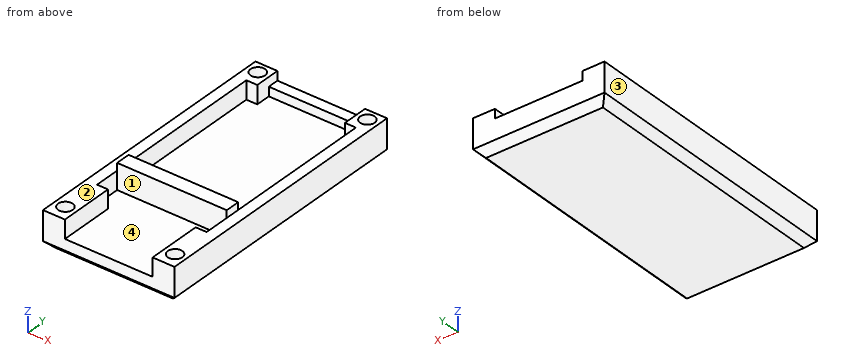
```python
from build123d import *

# Parameters (mm, degrees)
F1_DEPTH  = 37
F2_W      = 12
F2_H      = 1.25
F3_DEPTH  = 2
F5_DEPTH  = 2.5
F7_W      = 15
F7_H      = 2
F8_DEPTH  = 3.5
F9_R      = 1
F9_R_2    = 0.9349601775
F10_DEPTH = 2
F11_SIZE  = 1


with BuildPart() as f1:
    # F0 (on Front) → F1 (new body)
    with BuildSketch(Plane.XZ):
        Polygon((-9, 1), (-8, 0), (8, 0), (9, 1), (9, 5), (6, 5), (6, 2.5), (-6, 2.5), (-6, 5), (-9, 5), align=None)
    extrude(amount=F1_DEPTH)

    # F2 (on face) → F3 (join)
    with BuildSketch(Plane(origin=(0, 0, 0), x_dir=(-1, 0, 0), z_dir=(0, 1, 0))):
        with Locations((0, 3.125)):
            Rectangle(F2_W, F2_H)
    extrude(amount=-F3_DEPTH)

    # F4 (on face) → F5 (cut, through all)
    with BuildSketch(Plane.XY.offset(5)):
        Polygon((-7.5, -3.5), (-7.5, -29.5), (-6, -29.5), (-6, -35.5), (6, -35.5), (6, -29.5), (7.5, -29.5), (7.5, -3.5), (6, -3.5), (6, -1.5), (-6, -1.5), (-6, -3.5), align=None)
    extrude(amount=-F5_DEPTH, mode=Mode.SUBTRACT)

    # F7 (on offset) → F8 (join, through all)
    with BuildSketch(Plane.XY.offset(6)):
        with Locations((0, -25)):
            Rectangle(F7_W, F7_H)
    extrude(amount=-F8_DEPTH)

    # F9 (on face) → F10 (cut)
    with BuildSketch(Plane.XY.offset(5)):
        with Locations((-7.5, -35)):
            Circle(F9_R)
        with Locations((134.6376875191, -34.7655261621)):
            Circle(F9_R_2)
        with Locations((7.5, -35)):
            Circle(F9_R)
        with Locations((-7.5, -1.5)):
            Circle(F9_R)
        with Locations((7.5, -1.5)):
            Circle(F9_R)
    extrude(amount=-F10_DEPTH, mode=Mode.SUBTRACT)

    # F11
    f11_edges = [f1.edges().sort_by_distance(p)[0] for p in [
        (0, 0, 0),
        (0, -37, 0),
    ]]
    chamfer(f11_edges, length=F11_SIZE)


solid = f1.part
```
Build history of the part. All positions in model axes, mm. Face numbers are marked on the shaded views. Round coordinates to 2 decimals unless told otherwise and drop trailing zeros. Order: outer loops, then holes, each group sorted by start corner. A loop starts at its lowest first (then second) coordinate and runs counter-clockwise, first axis right, second up. Notation, with made-up numbers: (1.25, 30) -> (39.25, 30) arc R17 ccw to (39.25, 46) -> close; hole circle Ø1 at (0, -1.75). An arc over 180 degrees is marked (long way). Answer in a Markdown table with one row per item.
1) Mould opens along X. For the marked faces 1, 2, 3 and 4 say: released by +X, released by -X, zero draft, split by the parting line, or undercut.
Values:
| item | result |
|---|---|
| face 1 | undercut |
| face 2 | zero draft |
| face 3 | released by -X |
| face 4 | undercut |
2) Band-saw the part on B-B on x = 1.25. Give the cut face in (y, z).
Values:
| item | result |
|---|---|
| outline | (-37, 1) -> (-36, 0) -> (-1, 0) -> (0, 1) -> (0, 3.75) -> (-1.5, 3.75) -> (-1.5, 2.5) -> (-24, 2.5) -> (-24, 6) -> (-26, 6) -> (-26, 2.5) -> (-37, 2.5) -> close |
3) Pin check, flat tips, straight feed: P1, Ø1.6, axis at x = 7.5, y = -35, coming from the +Z side; P2, Ø2, axis at x = 7, y = -35, coming from the +Z side; P3, Ø1, axis at x = -3, z = 4.5, coming from the +Y side. Stop position of each tip, or through.
Values:
| item | result |
|---|---|
| P1 | z = 3 |
| P2 | z = 5 |
| P3 | y = -24 |
4) Wall check: L1, parallel to Z at x = 2, y = -22.5; L2, parallel to X at y = -20.5, z = 2.75; L3, parallel to Y at x = -4, z = 3.25. Give the ranges that are in metal, low to high.
Values:
| item | result |
|---|---|
| L1 | 0 to 2.5 |
| L2 | -9 to -7.5, 7.5 to 9 |
| L3 | -26 to -24, -1.5 to 0 |
5) Band-saw the part on A-A on y = -35. Give the cut face in (x, z).
Values:
| item | result |
|---|---|
| outline | (-9, 1) -> (-8, 0) -> (8, 0) -> (9, 1) -> (9, 5) -> (8.5, 5) -> (8.5, 3) -> (6.5, 3) -> (6.5, 5) -> (6, 5) -> (6, 2.5) -> (-6, 2.5) -> (-6, 5) -> (-6.5, 5) -> (-6.5, 3) -> (-8.5, 3) -> (-8.5, 5) -> (-9, 5) -> close |
6) Band-saw the part on C-C on y = -29. Give the cut face in (x, z), and give its area (3 significant figures).
Values:
| item | result |
|---|---|
| outline | (-9, 1) -> (-8, 0) -> (8, 0) -> (9, 1) -> (9, 5) -> (7.5, 5) -> (7.5, 2.5) -> (-7.5, 2.5) -> (-7.5, 5) -> (-9, 5) -> close |
| area | 51.5 mm2 |
